Can you work these out from the model? Positions are in its coordinate system, mm. A direction names the side the tool comes from. Round coordinates to 2 decimals unless told otherwise and drop trailing zeros. Order: outer loops, then holes, each group sorted by start corner. A loop starts at its lowest first (then second) coordinate and runs counter-clockwise, first axis right, second up.
Q1. If we section it at C-C (y = -1): Please give me the cut outline in (x, z).
Q2. If we section it at D-D (x = 17): Please give me the cut outline in (y, z), plus the area to 3 significant figures.
Q3. We'd pull the mould along X, two halves only. Please class faces 1 (the face through (-2, -12.472, 3)), 2 (the face through (37.25, -5, 3)), 3 (the face through (-3, -5, 3)): pulls with the +X half, pulls with the -X half, needs draft (parallel to the pull), parting line crosses it, or undercut.
Q4. For faces 4 (the face through (19, 1, 6.35)), 5 (the face through (39, -6.123, 3)), 6 (the face through (-1, -1, 3)), 7 (the face through (38.5, -3.3, 0)), which set-ups out of +Z, -Z, +X, -X, +Y, -Y let a thin tool reach every point of the face, with its end or its side?
Q5. Will these pins go through, and if not, where does the flat tip stop? P1, Ø0.8, axis at x = 39, z = 2, coming from the -Y side; P2, Ø3.5, axis at x = 36.5, y = -6.5, coming from the -Z side; P3, Ø1.5, axis at y = -2, z = -4, coming from the -X side; P4, Ø1.5, axis at x = 15.5, z = 3, coming from the -Y side.
Q6. If we section it at B-B (z = 5.25): Please give me the cut outline in (x, y).
Q7. If we section it at A-A (y = -3.5): Please give me the cut outline in (x, z).
Q8. If I drill on line 1 (Y direction, x = 1.5, z = 3); line 2 (X direction, y = -11.5, z = 1.75); line 3 (Z direction, x = 40, y = 2), over which ranges is the centre line in solid material (lowest first)?
from build123d import *

# Parameters (mm, degrees)
SKETCH2_W                           = 2.75
SKETCH2_H                           = 3.07
BOSS_EXTRUDE2_DEPTH                 = 6.35
SKETCH3_W                           = 23
SKETCH3_H                           = 6.35
BOSS_EXTRUDE3_DEPTH                 = 2
F_4_40_TAPPED_HOLE1_D               = 2.2606
F_4_40_TAPPED_HOLE1_DEPTH           = 3.91
F_4_40_TAPPED_HOLE1_TIP             = 0.679152758
F_4_40_TAPPED_HOLE1_ON_FACE_2_D     = 2.2606
F_4_40_TAPPED_HOLE1_ON_FACE_2_DEPTH = 3.91
F_4_40_TAPPED_HOLE1_ON_FACE_2_TIP   = 0.679152758
FILLET1_R                           = 1


with BuildPart() as part:
    # Sketch2 → Boss-Extrude2 (new body)
    with BuildSketch(Plane.XY):
        Polygon((-3, -12.4725), (-1, -12.4725), (-1, -6.1225), (-1, -3.0525), (-1, 0.5), (40, 0.5), (40, -3.0525), (40, -6.1225), (40, -12.4725), (42, -12.4725), (42, 2.5), (-3, 2.5), align=None)
        with Locations((0.375, -4.5875)):
            Rectangle(SKETCH2_W, SKETCH2_H)
        with Locations((38.625, -4.5875)):
            Rectangle(SKETCH2_W, SKETCH2_H)
    extrude(amount=BOSS_EXTRUDE2_DEPTH)

    # Sketch3 → Boss-Extrude3 (add)
    with BuildSketch(Plane(origin=(0, 2.5, 0), x_dir=(1, 0, 0), z_dir=(0, 1, 0))):
        with Locations((19.5, 3.175)):
            Rectangle(SKETCH3_W, SKETCH3_H)
    extrude(amount=-BOSS_EXTRUDE3_DEPTH)

    # #4-40 Tapped Hole1
    with Locations(Plane(origin=(-3, -9.1225, 3.175), x_dir=(0, -1, 0), z_dir=(-1, 0, 0))):
        with Locations((0, 0)):
            Hole(F_4_40_TAPPED_HOLE1_D / 2, depth=F_4_40_TAPPED_HOLE1_DEPTH)
            with Locations((0, 0, -(F_4_40_TAPPED_HOLE1_DEPTH + F_4_40_TAPPED_HOLE1_TIP / 2))):  # 118° drill point
                Cone(0, F_4_40_TAPPED_HOLE1_D / 2, F_4_40_TAPPED_HOLE1_TIP, mode=Mode.SUBTRACT)

    # #4-40 Tapped Hole1 on face 2
    with Locations(Plane(origin=(42, -9.1225, 3.175), x_dir=(0, 0, 1), z_dir=(1, 0, 0))):
        with Locations((0, 0)):
            Hole(F_4_40_TAPPED_HOLE1_ON_FACE_2_D / 2, depth=F_4_40_TAPPED_HOLE1_ON_FACE_2_DEPTH)
            with Locations((0, 0, -(F_4_40_TAPPED_HOLE1_ON_FACE_2_DEPTH + F_4_40_TAPPED_HOLE1_ON_FACE_2_TIP / 2))):  # 118° drill point
                Cone(0, F_4_40_TAPPED_HOLE1_ON_FACE_2_D / 2, F_4_40_TAPPED_HOLE1_ON_FACE_2_TIP, mode=Mode.SUBTRACT)

    # Fillet1
    fillet1_edges = [part.edges().sort_by_distance(p)[0] for p in [
        (40, 0.5, 3.175),
        (-1, 0.5, 3.175),
        (-1, -3.0525, 3.175),
        (40, -3.0525, 3.175),
    ]]
    fillet(fillet1_edges, radius=FILLET1_R)


solid = part.part
Solution:
1. outline: (-3, 0) - (-1, 0) - (-1, 6.35) - (-3, 6.35) - close; (40, 0) - (42, 0) - (42, 6.35) - (40, 6.35) - close
2. outline: (0.5, -6.35) - (2.5, -6.35) - (2.5, 6.35) - (0.5, 6.35) - close
2. area: 25.4 mm2
3. face 1: needs draft
3. face 2: undercut
3. face 3: pulls with the -X half
4. face 4: +Z, +X, -X, +Y, -Y
4. face 5: +Z, -Z, -Y
4. face 6: +Z, -Z
4. face 7: -Z, +X, +Y, -Y
5. P1: stops at y = -6.12
5. P2: stops at z = 0
5. P3: passes through
5. P4: stops at y = 0.5
6. outline: (-3, -12.47) - (-1, -12.47) - (-1, -6.12) - (1.75, -6.12) - (1.75, -3.05) - (0, -3.05) arc R1 cw to (-1, -2.05) - (-1, -0.5) arc R1 cw to (0, 0.5) - (39, 0.5) arc R1 cw to (40, -0.5) - (40, -2.05) arc R1 cw to (39, -3.05) - (37.25, -3.05) - (37.25, -6.12) - (40, -6.12) - (40, -12.47) - (42, -12.47) - (42, 2.5) - (-3, 2.5) - close
7. outline: (-3, 0) - (1.75, 0) - (1.75, 6.35) - (-3, 6.35) - close; (37.25, 0) - (42, 0) - (42, 6.35) - (37.25, 6.35) - close
8. line 1: y = -6.12 to -3.05, 0.5 to 2.5
8. line 2: x = -3 to -1, 40 to 42
8. line 3: z = 0 to 6.35
